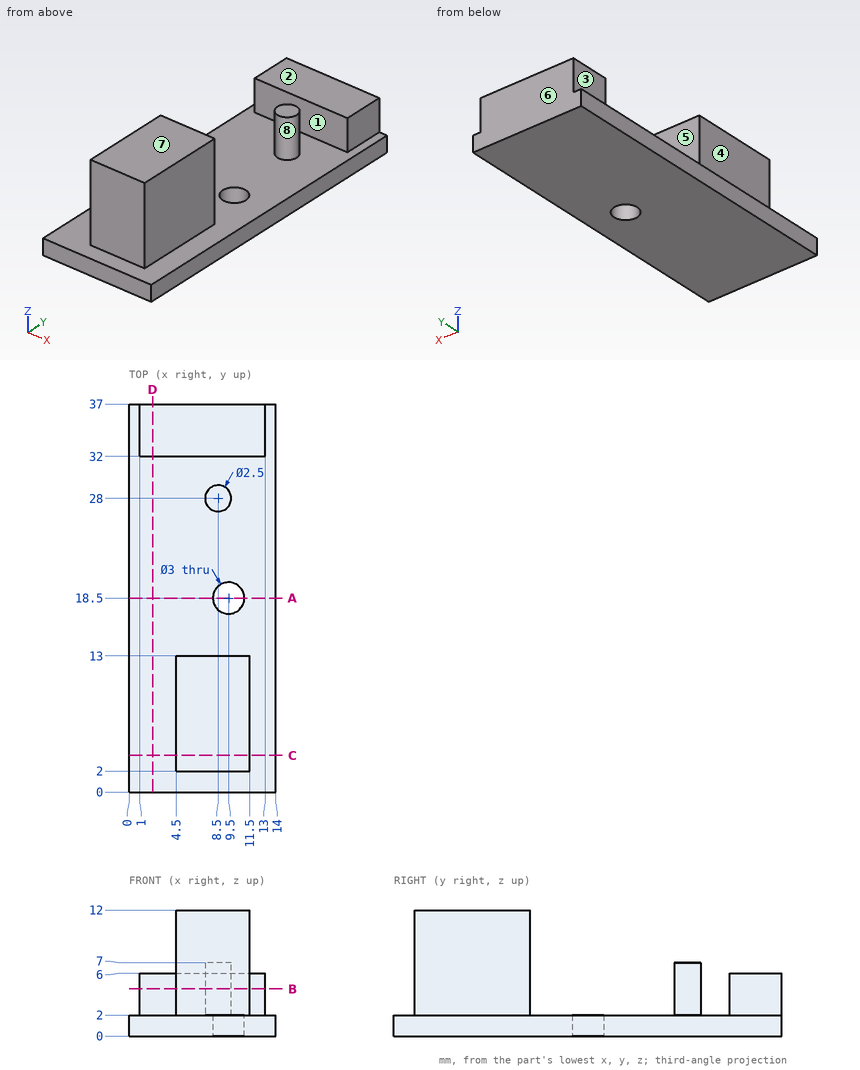
Verification items for this drawing (mm, ordinates from the low corner). A direction names the side the tool comes from. Round coordinates to 2 decimals unless told otherwise and drop trailing zeros. Write each loop counter-clockwise with the first axis right and the second up, starting at its lowest first coordinate (ties: lowest second). Pieces come first, ordered by that corner, then holes. Notation, with made-up numbers: M 56,84.5 L 107,84.5 A19 cw 107,100.5 Z; hole C 61.25,0 d6. An arc over 180 degrees is marked long. Write item = value, one per line. Start each with the question number.
1. Section check B-B, the plane z = 4.5. Record the cut outline in (x, y).
2. Section check A-A, the plane y = 18.5. Record the cut outline in (x, z).
3. Release check for a two-part mould opening along Y. For the marked faces 5, 6, 7 and 8 record: pulls with the +Y half, pulls with the -Y half, needs draft (parallel to the pull), parting line crosses it, or undercut.
4. Section check C-C, the plane y = 3.5. Record the cut outline in (x, z), then the cut area to 3 significant figures.
5. Section check D-D, the plane x = 2.25. Record the cut outline in (y, z), then the cut area to 3 significant figures.
6. Tool access check on the marked faces 1, 2, 3 and 4. Record the directions out of +Z, -Z, +X, -X, +Y, -Y that give a thin tool (end or side, any length) a straight path to the whole face; none if there is none.
7. Gauge pin test, flat ends, axial feed: pin 1 (3 mm diameter, centred on x = 2, y = 5, fed in from +Z); pin 2 (1 mm diameter, centred on y = 32.5, z = 5.5, fed in from +X); pin 3 (5 mm diameter, centred on y = 6, z = 6, fed in from +X). Record the tip position at first contact, or that the pin passes through.
8. Scan lines: line 1 (Y direction, x = 10, z = 5.25); line 2 (Y direction, x = 9.5, z = 0.65); line 3 (X direction, y = 9, z = 11.25). Record each from-to range of solid material in increasing order. Write a range as [from, to].
Results found:
q1.outline = M 1,32 L 13,32 L 13,37 L 1,37 Z; M 4.5,2 L 11.5,2 L 11.5,13 L 4.5,13 Z; C 8.5,28 d2.5
q2.outline = M 0,0 L 8,0 L 8,2 L 0,2 Z; M 11,0 L 14,0 L 14,2 L 11,2 Z
q3.face_5 = undercut
q3.face_6 = pulls with the +Y half
q3.face_7 = needs draft
q3.face_8 = undercut
q4.outline = M 0,0 L 14,0 L 14,2 L 11.5,2 L 11.5,12 L 4.5,12 L 4.5,2 L 0,2 Z
q4.area = 98.0 mm^2
q5.outline = M 0,0 L 37,0 L 37,6 L 32,6 L 32,2 L 0,2 Z
q5.area = 94.0 mm^2
q6.face_1 = +Z, +X, -X
q6.face_2 = +Z, +X, -X, +Y
q6.face_3 = +Z, -X, +Y, -Y
q6.face_4 = +Z, -X, -Y
q7.pin_1 = 2
q7.pin_2 = 13
q7.pin_3 = 11.5
q8.line_1 = [2, 13], [32, 37]
q8.line_2 = [0, 17], [20, 37]
q8.line_3 = [4.5, 11.5]
